Here's how the part is built. I have some questions about the finished solid (model axes, mm). A direction names the side the tool comes from. Give positions to 0.01 mm unless a question says otherwise; leave off trailing zeros. Loops run counter-clockwise (first coordinate to the right, second up) from the corner with the lowest first, then second, coordinate; pieces in that order, holes last. Notation, with made-up numbers: (67.5, 33) - (109.5, 33) arc R23 ccw to (109.5, 63) - close; hole circle Ø3 at (74, 46.25). An arc over 180 degrees is marked (long way). Return JSON: item names as keys, results as strings. Group by question number.
(1) If we mould it in two halves opening along X, with no side actions, what happens to faces 3 (the cylindrical face through (1.5, -11.4, 9.4)), 4 (the cylindrical face through (-8.63, -2.72, 11.05)), 5 (the flat face through (-2, 9, 0))? For each: released by +X, released by -X, zero draft, split by the parting line, or undercut.
(2) For P1, Ø1, axis at y = 7, z = 3, coming from the -X side; P2, Ø6, axis at y = 2, z = 5.5, coming from the -X side; P3, Ø4, axis at x = 4, z = 3.5, coming from the +Y side; P4, Ø14.5, axis at x = 0, y = 0, coming from the -Z side, each with a flat end and sliding along its axis, tell me the tip position at first contact or that it passes through.
(3) On a 3-axis mill with a long thin cutter (end or side, diameter ignored), from which of +Z, -Z, +X, -X, +Y, -Y can I reach the whole of each face in a straight line? I mean faces 1 (the flat face through (6.3, 10.3, 18.8)), 2 (the flat face through (9, 3, 21.8)). Say none if no direction works.
(4) If we section it at D-D (y = 12.25): Please give me the cut outline in (x, z).
(5) If we section it at C-C (z = 12): Please give me the cut outline in (x, y).
(6) I need wall thicknesses on probe 1 along Y at (x, z) = (0, 7.5); probe 2 along X at (y, z) = (4.5, 7). Which ranges of each line are inside material? Lowest first, please. Write a range as [from, to].
(7) If we section it at A-A (x = 0): Please give me the cut outline in (y, z), then the cut area to 3 significant figures.
```python
from build123d import *

# Parameters (mm, degrees)
F4_R    = 0.3
F5_SIZE = 0.5


with BuildPart() as f3:
    # F2 (on Front) → F3 (revolve)
    with BuildSketch(Plane.XZ):
        Polygon((-9.05, 21.8), (-14, 21.8), (-14, 18.8), (-11.5, 18.8), (-11.5, 0), (-9.05, 0), align=None)
    revolve(axis=Axis((0, 0, 10.9), (0, 0, 1)))

    # F4
    f4_edges = [f3.edges().sort_by_distance(p)[0] for p in [
        (11.5, 0, 18.8),
    ]]
    fillet(f4_edges, radius=F4_R)

    # F5
    f5_edges = [f3.edges().sort_by_distance(p)[0] for p in [
        (11.5, 0, 0),
    ]]
    chamfer(f5_edges, length=F5_SIZE)


solid = f3.part
```
Values:
{
 "1": {"face 3": "split by the parting line", "face 4": "undercut", "face 5": "zero draft"},
 "2": {"P1": "x = -9.49", "P2": "x = -11.5", "P3": "y = 11.32", "P4": "through"},
 "3": {"face 1": "-Z", "face 2": "+Z, +X, -X, +Y, -Y"},
 "4": {"outline": "(-6.78, 18.8) - (6.78, 18.8) - (6.78, 21.8) - (-6.78, 21.8) - close"},
 "5": {"outline": "circle Ø23 at (0, 0); hole circle Ø18.1 at (0, 0)"},
 "6": {"probe 1": "[-11.5, -9.05], [9.05, 11.5]", "probe 2": "[-10.58, -7.85], [7.85, 10.58]"},
 "7": {"outline": "(-14, 18.8) - (-11.8, 18.8) arc R0.3 cw to (-11.5, 18.5) - (-11.5, 0.5) - (-11, 0) - (-9.05, 0) - (-9.05, 21.8) - (-14, 21.8) - close; (9.05, 0) - (11, 0) - (11.5, 0.5) - (11.5, 18.5) arc R0.3 cw to (11.8, 18.8) - (14, 18.8) - (14, 21.8) - (9.05, 21.8) - close", "area": "122 mm2"}
}
